Could you check a few things on this model? Use its own coordinates, in mm. A direction names the side the tool comes from. Coordinates: 2 decimals unless noted, no trailing zeros. Order: outer loops, then holes, each group sorted by start corner. A loop starts at its lowest first (then second) coordinate and runs counter-clockwise, first axis right, second up. Notation, with made-up numbers: (27, -20) - (69, -20) arc R23 ccw to (69, 0) - close; hole circle Ø9 at (72, -2.75). An arc over 180 degrees is marked (long way). Answer as CSV lines item,"result". Start each with the question number.
1. For pin 1 (1.9 mm diameter, centred on y = 19, z = 4.5, fed in from +X); pin 2 (1.5 mm diameter, centred on y = 9, z = 4.5, fed in from -X); pin 3 (3 mm diameter, centred on y = 19.5, z = 4.5, fed in from -X); pin 4 (8 mm diameter, centred on x = -35, y = 18, fed in from +Z), each with a flat end and sliding along its axis, tell me the tip position at first contact or that it passes through.
2. I want a section at D-D, the plane x = -8. List the corners of the cut face in (y, z) for me, and give its area (3 significant figures).
3. Thinking about a two-plate mould opening in Y: for faces 6 (the face through (-40.314, -3.551, 3.131)), 7 (the face through (-15, 0, 0)), 8 (the face through (-29, -18.98, 3.13)), which applies, released by +Y, released by -Y, zero draft, split by the parting line, or undercut?
4. I want a section at A-A, the plane y = 0. List the corners of the cut face in (x, z) for me (3 decimals), and give its area (3 significant figures).
5. For faces 1 (the face through (12.7, 12, 3)), 2 (the face through (-6.35, -21, 3)), 3 (the face through (-12.802, 12, 3)), 4 (the face through (-19.152, 12, 3)), 5 (the face through (6.35, -21, 3)), which set-ups out of +Z, -Z, +X, -X, +Y, -Y let a thin tool reach every point of the face, with its end or its side?
6. I want a section at C-C, the plane x = -31.75. List the corners of the cut face in (y, z) for me, and give its area (3 significant figures).
7. I need wall thicknesses on probe 1 along Y at (x, z) = (-34.5, 4); probe 2 along X at (y, z) = (1, 4); probe 3 along Y at (x, z) = (-28, 5.25). Which ranges of each line are inside material? Lowest first, please.
from build123d import *

# Parameters (mm, degrees)
MASS_DEPTH          = 6.35
SKETCH4_R           = 9.271
CUT_EXTRUDE1_DEPTH  = 54.623672769
SKETCH3_W           = 12.7
SKETCH3_H           = 12.7
CUT_EXTRUDE2_DEPTH  = 54.623672769
LPATTERN1_COUNT     = 2
LPATTERN1_PITCH     = 25.4
CAVITY1_START       = -19.1516
CAVITY1_OUTLINE_W   = 11.1125
CAVITY1_OUTLINE_H   = 6.35
CAVITY1_DEPTH       = 6.35
CAVITY1_START_2     = 12.7
CAVITY1_2_OUTLINE_W = 11.1125
CAVITY1_2_OUTLINE_H = 6.35
CAVITY1_2_DEPTH     = 6.35


# Read off the part's stored shape, not the designer's step: Cavity1
with BuildPart() as part:
    # Sketch1 → Mass (new body)
    with BuildSketch(Plane.XY):
        with BuildLine():
            Line((-19.05, -23.8125), (19.05, -23.8125))
            Line((19.05, -23.8125), (19.05, 23.8125))
            Line((19.05, 23.8125), (-19.05, 23.8125))
            Line((-19.05, 23.8125), (-38.68314018, 14.281008096))
            ThreePointArc((-38.68314018, 14.281008096), (-47.625, 0), (-38.68314018, -14.281008096))
            Line((-38.68314018, -14.281008096), (-19.05, -23.8125))
        make_face()
    extrude(amount=MASS_DEPTH)

    # Sketch4 → Cut-Extrude1 (cut, through all)
    with BuildSketch(Plane(origin=(0, 0, 0), x_dir=(-1, 0, 0), z_dir=(0, 0, -1))):
        with Locations((31.75, 0)):
            Circle(SKETCH4_R)
    extrude(amount=-CUT_EXTRUDE1_DEPTH, mode=Mode.SUBTRACT)

    # Sketch3 → Cut-Extrude2 (cut, through all)
    with BuildSketch(Plane(origin=(0, 0, 0), x_dir=(-1, 0, 0), z_dir=(0, 0, -1))):
        with Locations((-12.7, 23.8125)):
            Rectangle(SKETCH3_W, SKETCH3_H)
        with Locations((-12.7, -23.8125)):
            Rectangle(SKETCH3_W, SKETCH3_H)
    cut_extrude2 = extrude(amount=-CUT_EXTRUDE2_DEPTH, mode=Mode.SUBTRACT)

    # LPattern1: Cut-Extrude2 ×2
    with Locations(*[(-i * LPATTERN1_PITCH, 0, 0) for i in range(1, LPATTERN1_COUNT)]):
        add(cut_extrude2, mode=Mode.SUBTRACT)

    # Cavity1 outline → Cavity1 (cut)
    with BuildSketch(Plane.YZ.offset(CAVITY1_START)):
        with Locations((-11.90625, 3.175)):
            Rectangle(CAVITY1_OUTLINE_W, CAVITY1_OUTLINE_H)
        with Locations((11.90625, 3.175)):
            Rectangle(CAVITY1_OUTLINE_W, CAVITY1_OUTLINE_H)
    extrude(amount=CAVITY1_DEPTH, mode=Mode.SUBTRACT)

    # Cavity1 2 outline → Cavity1 2 (cut)
    with BuildSketch(Plane.YZ.offset(CAVITY1_START_2)):
        with Locations((-11.90625, 3.175)):
            Rectangle(CAVITY1_2_OUTLINE_W, CAVITY1_2_OUTLINE_H)
        with Locations((11.90625, 3.175)):
            Rectangle(CAVITY1_2_OUTLINE_W, CAVITY1_2_OUTLINE_H)
    extrude(amount=CAVITY1_2_DEPTH, mode=Mode.SUBTRACT)


solid = part.part
Solved:
1,pin 1,"stops at x = 6.35"
1,pin 2,"stops at x = -45.31"
1,pin 3,"stops at x = -31.02"
1,pin 4,"stops at z = 6.35"
2,outline,"(-17.46, 0) - (17.46, 0) - (17.46, 6.35) - (-17.46, 6.35) - close"
2,area,"222 mm2"
3,face 6,"undercut"
3,face 7,"zero draft"
3,face 8,"released by -Y"
4,outline,"(-47.625, 0) - (-41.021, 0) - (-41.021, 6.35) - (-47.625, 6.35) - close; (-22.479, 0) - (19.05, 0) - (19.05, 6.35) - (-22.479, 6.35) - close"
4,area,"306 mm2"
5,face 1,"+Z, -Z, +X, +Y"
5,face 2,"+Z, -Z, -Y"
5,face 3,"+Z, -Z, +Y"
5,face 4,"+Z, -Z"
5,face 5,"+Z, -Z, +X, -Y"
6,outline,"(-17.65, 0) - (-9.27, 0) - (-9.27, 6.35) - (-17.65, 6.35) - close; (9.27, 0) - (17.65, 0) - (17.65, 6.35) - (9.27, 6.35) - close"
6,area,"106 mm2"
7,probe 1,"y = -16.31 to -8.85, 8.85 to 16.31"
7,probe 2,"x = -47.59 to -40.97, -22.53 to 19.05"
7,probe 3,"y = -19.47 to -8.48, 8.48 to 19.47"
